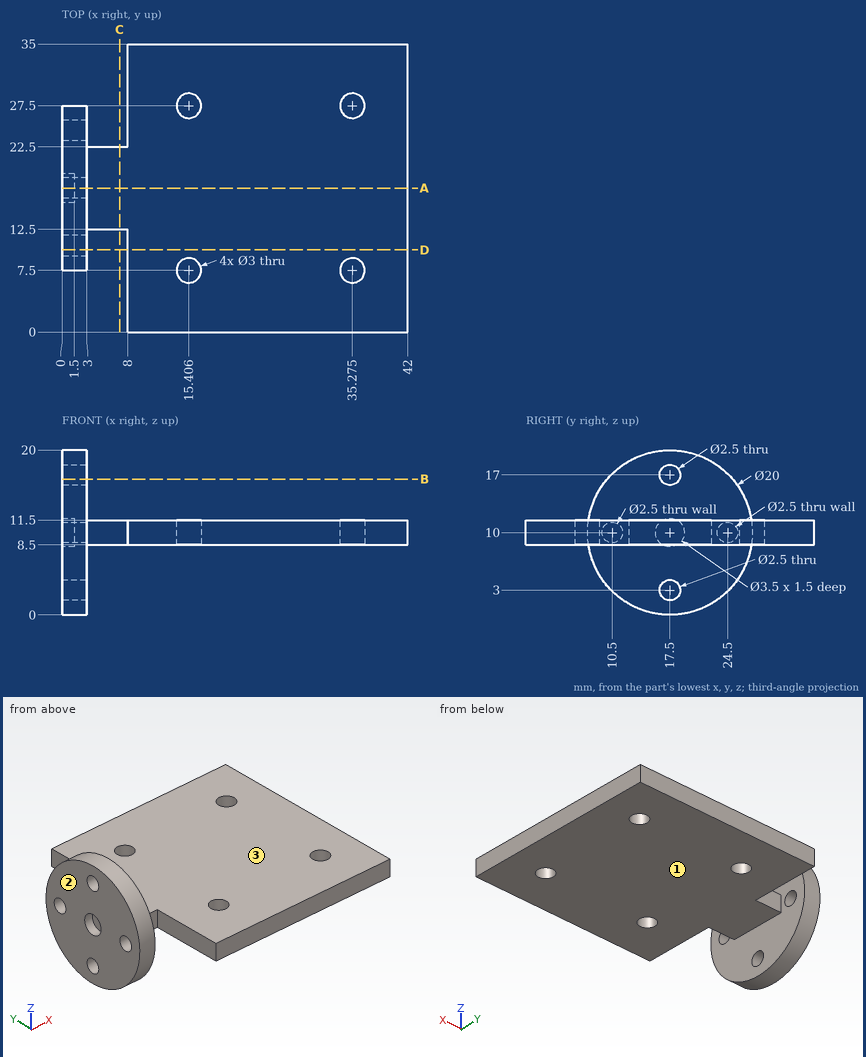
Could you check a few things on this drawing? It's one solid part, dimensions in mm from its lowest x, y, z. A direction names the side the tool comes from. Round coordinates to 2 decimals unless told otherwise and drop trailing zeros. Write each loop counter-clockwise with the first axis right and the second up, starting at its lowest first coordinate (ties: lowest second). Pieces come first, ordered by that corner, then holes. Notation, with made-up numbers: (-2.5, 72.5) -> (27.5, 72.5) arc R33 cw to (27.5, 104.5) -> close; hole circle Ø6 at (61, 79). An arc over 180 degrees is marked (long way). One line per item, written item: value.
1) Suppose I cut it at C-C on x = 7. List the corners of the cut face in (y, z) for me.
Filled sheet:
outline: (12.5, 8.5) -> (22.5, 8.5) -> (22.5, 11.5) -> (12.5, 11.5) -> close
2) Suppose I cut it at D-D on y = 10. List the corners of the cut face in (x, z) for me (1 decimal), plus the area to 3 significant figures.
Filled sheet:
outline: (0, 3.4) -> (3, 3.4) -> (3, 8.9) -> (0, 8.9) -> close; (0, 11.1) -> (3, 11.1) -> (3, 16.6) -> (0, 16.6) -> close; (8, 8.5) -> (42, 8.5) -> (42, 11.5) -> (8, 11.5) -> close
area: 135 mm2
3) If I drill on line 1 (Y direction, x = 0.6, z = 10); line 2 (Y direction, x = 1.55, z = 10); line 3 (X direction, y = 24, z = 13.5), over which ranges is the centre line in solid material (lowest first)? Write a range as [from, to].
Filled sheet:
line 1: y = [7.5, 9.25], [11.75, 15.75], [19.25, 23.25], [25.75, 27.5]
line 2: y = [7.5, 9.25], [11.75, 23.25], [25.75, 27.5]
line 3: x = [0, 3]
4) For the marked faces 1, 2 and 3, which set-ups out of +Z, -Z, +X, -X, +Y, -Y let a thin tool reach every point of the face, with its end or its side?
Filled sheet:
face 1: -Z, +X, +Y, -Y
face 2: +Z, -Z, -X, +Y, -Y
face 3: +Z, +X, +Y, -Y
5) Suppose I cut it at A-A on y = 17.5. List the corners of the cut face in (x, z) for me, plus the area to 3 significant figures.
Filled sheet:
outline: (0, 0) -> (3, 0) -> (3, 1.75) -> (0, 1.75) -> close; (0, 4.25) -> (3, 4.25) -> (3, 8.5) -> (42, 8.5) -> (42, 11.5) -> (3, 11.5) -> (3, 15.75) -> (0, 15.75) -> (0, 11.75) -> (1.5, 11.75) -> (1.5, 8.25) -> (0, 8.25) -> close; (0, 18.25) -> (3, 18.25) -> (3, 20) -> (0, 20) -> close
area: 157 mm2
6) I'm going to push flat-ended pins straight in: pin 1 Ø2 at (x, y) = (24.5, 31) entering from +Z; pin 2 Ø3.5 at (y, z) = (31, 9.5) entering from -X; pin 3 Ø3.5 at (x, y) = (35.28, 7.5) entering from -Z. Where does each tip first touch, or does it pass through?
Filled sheet:
pin 1: stops at z = 11.5
pin 2: stops at x = 8
pin 3: stops at z = 8.5
7) Suppose I cut it at B-B on z = 16.5. List the corners of the cut face in (x, y) for me (1 decimal).
Filled sheet:
outline: (0, 9.9) -> (3, 9.9) -> (3, 16.4) -> (0, 16.4) -> close; (0, 18.6) -> (3, 18.6) -> (3, 25.1) -> (0, 25.1) -> close
